Verification items for the finished model (mm, model axes). A direction names the side the tool comes from. Round coordinates to 2 decimals unless told otherwise and drop trailing zeros. Order: outer loops, then holes, each group sorted by start corner. A loop starts at its lowest first (then second) coordinate and runs counter-clockwise, first axis right, second up. Notation, with made-up numbers: (22.25, 68) -> (70.25, 68) arc R23 cw to (70.25, 92) -> close; hole circle Ø1 at (-24, 46.25). An arc over 180 degrees is marked (long way). Return JSON: item names as keys, results as strings. Group by question number.
1) Section check A-A on z = 5.5. State how many separate pieces and enclosed holes the cut face has, plus the area to 3 significant figures.
2) Tool access check on faces 1 (the flat face through (128, 60, 4)), 2 (the flat face through (137, 3, 3)), 3 (the flat face through (5, 10.5, 4)), 4 (the flat face through (7, 79, 3)). Record the directions out of +Z, -Z, +X, -X, +Y, -Y that give a thin tool (end or side, any length) a straight path to the whole face; none if there is none.
3) Section check D-D on y = 69.5. Enter the section's corners in (x, z).
4) Depth check by flat-ended pin: pin 1 (4 mm diameter, centred on y = 19.5, z = 4.5, fed in from +X); pin 2 (1 mm diameter, centred on y = 50.5, z = 5.5, fed in from +X); pin 3 (3.5 mm diameter, centred on y = 87.5, z = 5, fed in from -X). Enter the tip coordinate at first touch or a pass-through.
5) Scan lines: L1, parallel to X at y = 19, z = 5.75; L2, parallel to X at y = 61.5, z = 4; L3, parallel to X at y = 14, z = 4. Record each from-to range of solid material in increasing order.
6) Draft check along X on faces 5 (the flat face through (9, 59, 4)), 6 (the flat face through (68, 56, 0)), 7 (the flat face through (0, 3, 3)). Enter one of: pulls with the +X half, pulls with the -X half, needs draft (parallel to the pull), parting line crosses it, or undercut.
7) Section check C-C on x = 109.5. Enter the section's corners in (y, z).
8) Section check B-B on y = 96. Enter the section's corners in (x, z), plus the area to 3 significant figures.
```python
from build123d import *

# Parameters (mm, degrees)
F1_DEPTH = 2
F2_R     = 40
F3_R     = 60
F5_DEPTH = 5
F6_W     = 119
F6_H     = 20
F7_DEPTH = 2


with BuildPart() as f1:
    # F0 (on Top) → F1 (new body)
    with BuildSketch(Plane.XY):
        Polygon((0, 10.5), (0, 0), (68.5, 0), (137, 0), (137, 10.5), (130, 40.5), (130, 110.5), (68.5, 110.5), (7, 110.5), (7, 40.5), align=None)
    extrude(amount=F1_DEPTH)

    # F2
    f2_edges = [f1.edges().sort_by_distance(p)[0] for p in [
        (137, 10.5, 1),
        (0, 10.5, 1),
    ]]
    fillet(f2_edges, radius=F2_R)

    # F3
    f3_edges = [f1.edges().sort_by_distance(p)[0] for p in [
        (7, 40.5, 1),
        (130, 40.5, 1),
    ]]
    fillet(f3_edges, radius=F3_R)

    # F4 (on face) → F5 (join)
    with BuildSketch(Plane.XY.offset(2)):
        with BuildLine():
            Line((130, 110.5), (128, 110.5))
            Line((128, 110.5), (128, 47.40723087))
            Line((128, 47.40723087), (128, 8.5))
            Line((128, 8.5), (134.9106173749, 8.5))
            ThreePointArc((134.9106173749, 8.5), (134.9776477697, 7.1983562602), (135, 5.89517942))
            Line((135, 5.89517942), (135, 2))
            Line((135, 2), (128, 2))
            Line((128, 2), (128, 0))
            Line((128, 0), (137, 0))
            Line((137, 0), (137, 5.89517942))
            ThreePointArc((137, 5.89517942), (136.7375511046, 10.4697867481), (135.9536483897, 14.9843640443))
            Line((135.9536483897, 14.9843640443), (131.5695274155, 33.7734539336))
            ThreePointArc((131.5695274155, 33.7734539336), (130.393673343, 40.5453198778), (130, 47.40723087))
            Line((130, 47.40723087), (130, 110.5))
        make_face()
        with BuildLine():
            Line((134.7199632479, 10.5), (130, 10.5))
            Line((130, 10.5), (130, 31.6983303996))
            Line((130, 31.6983303996), (134.0059659702, 14.5299048131))
            ThreePointArc((134.0059659702, 14.5299048131), (134.4172574834, 12.5245717316), (134.7199632479, 10.5))
        make_face(mode=Mode.SUBTRACT)
        with BuildLine():
            Line((9, 8.5), (9, 47.40723087))
            Line((9, 47.40723087), (9, 110.5))
            Line((9, 110.5), (7, 110.5))
            Line((7, 110.5), (7, 47.40723087))
            ThreePointArc((7, 47.40723087), (6.606326657, 40.5453198778), (5.4304725845, 33.7734539336))
            Line((5.4304725845, 33.7734539336), (1.0463516103, 14.9843640443))
            ThreePointArc((1.0463516103, 14.9843640443), (0.2624488954, 10.4697867481), (0, 5.89517942))
            Line((0, 5.89517942), (0, 0))
            Line((0, 0), (9, 0))
            Line((9, 0), (9, 2))
            Line((9, 2), (2, 2))
            Line((2, 2), (2, 5.89517942))
            ThreePointArc((2, 5.89517942), (2.0223522303, 7.1983562602), (2.0893826251, 8.5))
            Line((2.0893826251, 8.5), (9, 8.5))
        make_face()
        with BuildLine():
            ThreePointArc((2.2800367521, 10.5), (2.5827425166, 12.5245717316), (2.9940340298, 14.5299048131))
            Line((2.9940340298, 14.5299048131), (7, 31.6983303996))
            Line((7, 31.6983303996), (7, 10.5))
            Line((7, 10.5), (2.2800367521, 10.5))
        make_face(mode=Mode.SUBTRACT)
    extrude(amount=F5_DEPTH)

    # F6 (on face) → F7 (join)
    with BuildSketch(Plane.XY.offset(2)):
        with Locations((68.5, 100.5)):
            Rectangle(F6_W, F6_H)
    extrude(amount=F7_DEPTH)


solid = f1.part
```
Check result:
{
 "1": {"separate pieces": "2", "enclosed holes": "2", "area": "606 mm^2"},
 "2": {"face 1": "+Z, -Y", "face 2": "+Z, -Z, +X, +Y, -Y", "face 3": "+Z", "face 4": "+Z, -Z, -X, +Y"},
 "3": {"outline": "(7, 0) -> (130, 0) -> (130, 7) -> (128, 7) -> (128, 2) -> (9, 2) -> (9, 7) -> (7, 7) -> close"},
 "4": {"pin 1": "x = 135.37", "pin 2": "x = 130", "pin 3": "x = 7"},
 "5": {"L1": "1.98 to 4.04, 7 to 9, 128 to 130, 132.96 to 135.02", "L2": "7 to 9, 128 to 130", "L3": "0.83 to 2.87, 7 to 9, 128 to 130, 134.13 to 136.17"},
 "6": {"face 5": "undercut", "face 6": "needs draft", "face 7": "pulls with the -X half"},
 "7": {"outline": "(0, 0) -> (110.5, 0) -> (110.5, 4) -> (90.5, 4) -> (90.5, 2) -> (0, 2) -> close"},
 "8": {"outline": "(7, 0) -> (130, 0) -> (130, 7) -> (128, 7) -> (128, 4) -> (9, 4) -> (9, 7) -> (7, 7) -> close", "area": "504 mm^2"}
}
